```python
from build123d import *

# Parameters (mm, degrees)
SKETCH1_R           = 2.5
BOSS_EXTRUDE1_DEPTH = 5
SKETCH2_R           = 1.5
SKETCH2_W           = 50
SKETCH2_H           = 50
CUT_EXTRUDE1_DEPTH  = 5
SKETCH3_W           = 250
SKETCH3_H           = 300
CUT_EXTRUDE2_DEPTH  = 10
SKETCH4_R           = 3
CUT_EXTRUDE3_DEPTH  = 10


with BuildPart() as part:
    # Sketch1 → Boss-Extrude1 (new body)
    with BuildSketch(Plane.XY):
        with BuildLine():
            Line((-123.5, 121.5), (-123.5, -121.5))
            ThreePointArc((-123.5, -121.5), (-122.914213562, -122.914213562), (-121.5, -123.5))
            Line((-121.5, -123.5), (121.5, -123.5))
            ThreePointArc((121.5, -123.5), (122.914213562, -122.914213562), (123.5, -121.5))
            Line((123.5, -121.5), (123.5, 121.5))
            ThreePointArc((123.5, 121.5), (122.914213562, 122.914213562), (121.5, 123.5))
            Line((121.5, 123.5), (-121.5, 123.5))
            ThreePointArc((-121.5, 123.5), (-122.914213562, 122.914213562), (-123.5, 121.5))
        make_face()
        with Locations((-118.5, 118.5)):
            Circle(SKETCH1_R, mode=Mode.SUBTRACT)
        with Locations((118.5, 118.5)):
            Circle(SKETCH1_R, mode=Mode.SUBTRACT)
        with Locations((118.5, -118.5)):
            Circle(SKETCH1_R, mode=Mode.SUBTRACT)
        with Locations((-118.5, -118.5)):
            Circle(SKETCH1_R, mode=Mode.SUBTRACT)
    extrude(amount=BOSS_EXTRUDE1_DEPTH)

    # Sketch2 → Cut-Extrude1 (cut)
    with BuildSketch(Plane(origin=(0, 0, 0), x_dir=(-1, 0, 0), z_dir=(0, 0, -1))):
        with Locations((28.284271247, 28.284271247)):
            Circle(SKETCH2_R)
        with Locations((28.284271247, -28.284271247)):
            Circle(SKETCH2_R)
        with Locations((-28.284271247, -28.284271247)):
            Circle(SKETCH2_R)
        with Locations((-28.284271247, 28.284271247)):
            Circle(SKETCH2_R)
        Rectangle(SKETCH2_W, SKETCH2_H)
    extrude(amount=-CUT_EXTRUDE1_DEPTH, mode=Mode.SUBTRACT)

    # Sketch3 → Cut-Extrude2 (cut)
    with BuildSketch(Plane(origin=(0, 0, 0), x_dir=(-1, 0, 0), z_dir=(0, 0, -1))):
        with Locations((45, 0)):
            Rectangle(SKETCH3_W, SKETCH3_H)
    extrude(amount=-CUT_EXTRUDE2_DEPTH, mode=Mode.SUBTRACT)

    # Sketch4 → Cut-Extrude3 (cut)
    with BuildSketch(Plane(origin=(0, 0, 0), x_dir=(-1, 0, 0), z_dir=(0, 0, -1))):
        with Locations((-93, 78.5)):
            Circle(SKETCH4_R)
        with Locations((-93, 108.5)):
            Circle(SKETCH4_R)
        with Locations((-93, -78.5)):
            Circle(SKETCH4_R)
        with Locations((-93, -108.5)):
            Circle(SKETCH4_R)
    extrude(amount=-CUT_EXTRUDE3_DEPTH, mode=Mode.SUBTRACT)


solid = part.part
```
Build history of the part. All positions in model axes, mm. Give positions to 0.01 mm unless a question says otherwise; leave off trailing zeros. Order: outer loops, then holes, each group sorted by start corner. A loop starts at its lowest first (then second) coordinate and runs counter-clockwise, first axis right, second up. Notation, with made-up numbers: M 24.5,-6.75 L 57.5,-6.75 A30 ccw 57.5,18.25 Z; hole C -27,13 d9. An arc over 180 degrees is marked long. Write item = value, one per line. Start each with the question number.
(1) Probe L1, parallel to Y at x = 93, z = 2.1; L2, parallel to X at y = 106.5, z = 1.5. List the from-to ranges inside material, lowest first. Write a range as [from, to].
(2) Slice it at C-C on y = 108.5. Write the cut outline in (x, z), plus the area to 4 significant figures.
(3) Pin check, flat tip, straight feed: pin 1 Ø3.5 at (x, y) = (93, -108.5) entering from -Z. Stop position of the tip, or through.
(4) Two-plate mould, pull along Y, no slides. Class faces 1 (the cylindrical face through (95.4, -80.3, 2.5)), 2 (the flat face through (101, 2, 0)), 3 (the flat face through (100, -123.5, 2)): released by +Y, released by -Y, zero draft, split by the parting line, or undercut.
(5) Slice it at B-B on x = 93. Write the cut outline in (y, z).
(6) Slice it at A-A on y = -118.5. Write the cut outline in (x, z), plus the area to 4 significant figures.
Responses:
q1.L1 = [-123.5, -111.5], [-105.5, -81.5], [-75.5, 75.5], [81.5, 105.5], [111.5, 123.5]
q1.L2 = [80, 90.76], [95.24, 123.5]
q2.outline = M 80,0 L 90,0 L 90,5 L 80,5 Z; M 96,0 L 123.5,0 L 123.5,5 L 96,5 Z
q2.area = 187.5 mm2
q3.pin_1 = through
q4.face_1 = undercut
q4.face_2 = zero draft
q4.face_3 = released by -Y
q5.outline = M -123.5,0 L -111.5,0 L -111.5,5 L -123.5,5 Z; M -105.5,0 L -81.5,0 L -81.5,5 L -105.5,5 Z; M -75.5,0 L 75.5,0 L 75.5,5 L -75.5,5 Z; M 81.5,0 L 105.5,0 L 105.5,5 L 81.5,5 Z; M 111.5,0 L 123.5,0 L 123.5,5 L 111.5,5 Z
q6.outline = M 80,0 L 116,0 L 116,5 L 80,5 Z; M 121,0 L 123.5,0 L 123.5,5 L 121,5 Z
q6.area = 192.5 mm2
